Geometry check sheet. Reference: drawing and pictorial views, mm from the part's lowest x, y, z. Give positions to 0.01 mm unless a question says otherwise; leave off trailing zeros. Loops run counter-clockwise (first coordinate to the right, second up) from the corner with the lowest first, then second, coordinate; pieces in that order, holes last. Notation, with made-up numbers: (73, 19.5) - (85, 19.5) arc R15 ccw to (85, 43.5) - close; hole circle Ø2 at (35.25, -33). An arc over 180 degrees is marked (long way). Answer in a Markdown table with one row per item. Add a question column.
(1) Go/stop test with flat-tipped pins: P1, Ø1.5, axis at y = 6, z = 8.5, coming from the -X side; P2, Ø1, axis at x = 3, z = 5.5, coming from the -Y side. Record where each tip stops, or that it passes through.
(2) Thickness scan on L1, parallel to X at y = 9.5, z = 2.5; L2, parallel to Y at x = 9, z = 2.25; L3, parallel to Y at x = 4, z = 2. Record the ranges inside material, lowest first.
(3) Draft check along Y on the marked faces 1, 2 and 3. Enter one of: released by +Y, released by -Y, zero draft, split by the parting line, or undercut.
(4) Sectioned sample at B-B on x = 4. Enter the section's corners in (y, z).
(5) Sectioned sample at A-A on z = 2. Enter the section's corners in (x, y), then the cut area to 3 significant figures.
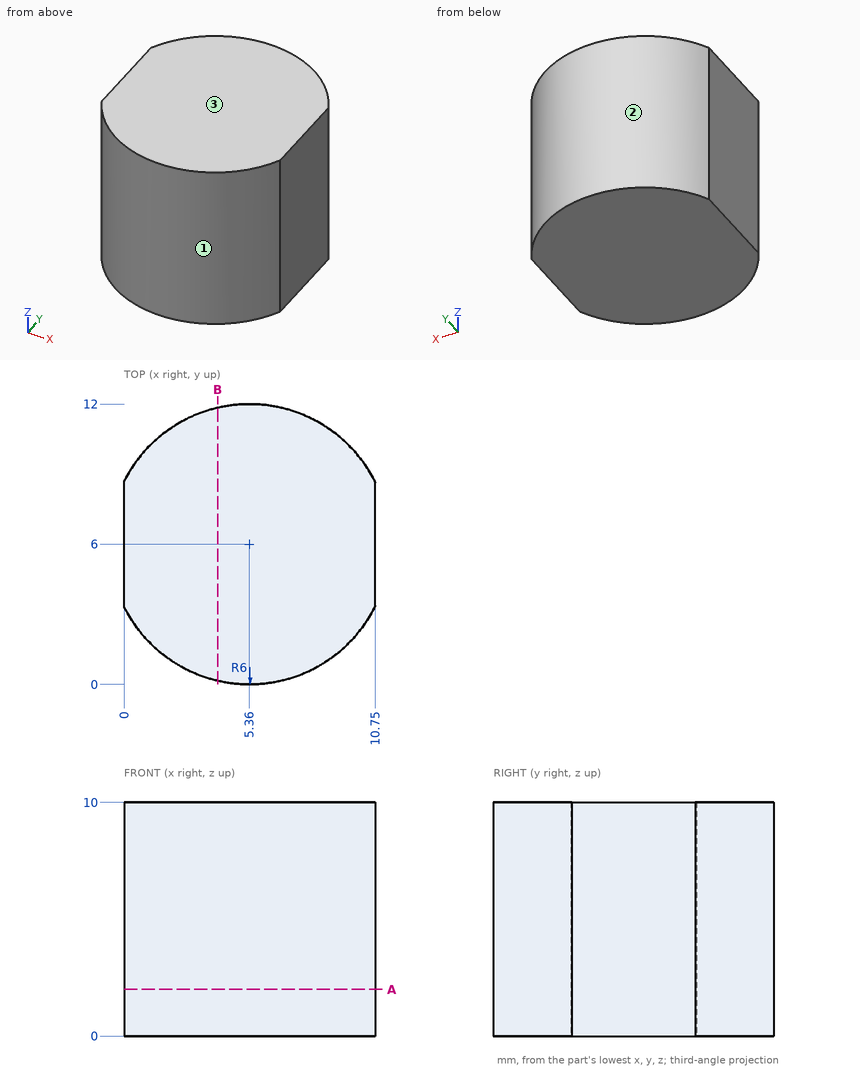
Reply:
| question | item | result |
|---|---|---|
| 1 | P1 | x = 0 |
| 1 | P2 | y = 0.3 |
| 2 | L1 | 0.49 to 10.23 |
| 2 | L2 | 1.23 to 10.77 |
| 2 | L3 | 0.16 to 11.84 |
| 3 | face 1 | released by -Y |
| 3 | face 2 | released by +Y |
| 3 | face 3 | zero draft |
| 4 | outline | (0.16, 0) - (11.84, 0) - (11.84, 10) - (0.16, 10) - close |
| 5 | outline | (0, 3.3) arc R6 ccw to (10.75, 3.36) - (10.75, 8.64) arc R6 ccw to (0, 8.7) - close |
| 5 | area | 109 mm^2 |
